```python
from build123d import *

# Parameters (mm, degrees)
SKETCH_W        = 10
SKETCH_H        = 15
PAD_DEPTH       = 220
SKETCH001_R     = 3
POCKET_DEPTH    = 15.001
SKETCH002_R     = 3.05
SKETCH002_R_2   = 1.55
POCKET001_DEPTH = 15.001
SKETCH003_R     = 1.5
POCKET002_DEPTH = 5
CHAMFER_SIZE    = 0.25


with BuildPart() as part:
    # Sketch → Pad (new body)
    with BuildSketch(Plane.XZ):
        with Locations((5, 7.5)):
            Rectangle(SKETCH_W, SKETCH_H)
    extrude(amount=PAD_DEPTH)

    # Sketch001 (on Face3 of Pad) → Pocket (cut, through all)
    with BuildSketch(Plane(origin=(0, 0, 15), x_dir=(-1, 0, 0), z_dir=(0, 0, 1))):
        with Locations((-5, 215)):
            Circle(SKETCH001_R)
        with Locations((-5, 145)):
            Circle(SKETCH001_R)
        with Locations((-5, 75)):
            Circle(SKETCH001_R)
        with Locations((-5, 5)):
            Circle(SKETCH001_R)
    extrude(amount=-POCKET_DEPTH, mode=Mode.SUBTRACT)

    # Sketch002 (on Face10 of Pocket) → Pocket001 (cut, through all)
    with BuildSketch(Plane(origin=(0, 0, 15), x_dir=(-1, 0, 0), z_dir=(0, 0, 1))):
        with Locations((-5, 130)):
            Circle(SKETCH002_R)
        with Locations((-5, 110)):
            Circle(SKETCH002_R_2)
        with Locations((-5, 90)):
            Circle(SKETCH002_R)
    extrude(amount=-POCKET001_DEPTH, mode=Mode.SUBTRACT)

    # Sketch003 (on Face2 of Pocket001) → Pocket002 (cut)
    with BuildSketch(Plane(origin=(0, 0, 0), x_dir=(0, 0, -1), z_dir=(-1, 0, 0))):
        with Locations((-7.5, 130)):
            Circle(SKETCH003_R)
        with Locations((-7.5, 110)):
            Circle(SKETCH003_R)
        with Locations((-7.5, 90)):
            Circle(SKETCH003_R)
    extrude(amount=-POCKET002_DEPTH, mode=Mode.SUBTRACT)

    # Chamfer
    chamfer_edges = [part.edges().sort_by_distance(p)[0] for p in [
        (0, -110, 15),
        (0, 0, 7.5),
        (0, -220, 7.5),
        (0, -110, 0),
        (0, -130, 9),
        (0, -110, 9),
        (0, -90, 9),
        (10, -110, 15),
        (5, 0, 15),
        (5, -220, 15),
        (8.05, -130, 15),
        (6.55, -110, 15),
        (8.05, -90, 15),
        (8, -75, 15),
        (8, -5, 15),
        (8, -215, 15),
        (8, -145, 15),
        (5, -220, 0),
        (10, -220, 7.5),
        (5, 0, 0),
        (10, -110, 0),
        (8.05, -130, 0),
        (6.55, -110, 0),
        (8.05, -90, 0),
        (8, -75, 0),
        (8, -5, 0),
        (8, -215, 0),
        (8, -145, 0),
        (10, 0, 7.5),
    ]]
    chamfer(chamfer_edges, length=CHAMFER_SIZE)


solid = part.part
```
Work out the finished part from the listing and answer in its coordinate system (mm). Round coordinates to 2 decimals unless told otherwise and drop trailing zeros. Loops run counter-clockwise (first coordinate to the right, second up) from the corner with the lowest first, then second, coordinate; pieces in that order, holes last. Notation, with made-up numbers: M 63.5,-21.5 L 102.5,-21.5 A14 cw 102.5,-14.5 Z; hole C -16,84.25 d6. An arc over 180 degrees is marked long. One line per question, with ' | ' between items.
Q1. The mould has two halves that part along X. Classify faces 1 (the cylindrical face through (3.616, -2.338, 7.602)), 2 (the flat face through (4, -108, 15)): +X half, -X half, draft (parallel to the pull), parting line (faces both ways), or undercut.
Conclusion:
face 1: undercut | face 2: draft
Q2. Consider line 1 along Y through (x, z) = (1.65, 7.5); line 2 along Z through (x, y) = (1.6, -90); line 3 along X through (y, z) = (-5, 9.75). Determine where each line is inside the solid, lowest interval first. Write a range as from..to.
Conclusion:
line 1: y = -220..-131.5, -128.5..-111.5, -108.5..-91.5, -88.5..0 | line 2: z = 0..6, 9..15 | line 3: x = 0..2, 8..10
Q3. Find section A-A, the plane z = 12.5. Give the vertices of the cut face in (x, y).
Conclusion:
outline: M 0,-219.75 L 0.25,-220 L 9.75,-220 L 10,-219.75 L 10,-0.25 L 9.75,0 L 0.25,0 L 0,-0.25 Z; hole C 5,-130 d6.1; hole C 5,-90 d6.1; hole C 5,-215 d6; hole C 5,-145 d6; hole C 5,-75 d6; hole C 5,-5 d6; hole C 5,-110 d3.1
